from build123d import *

# Parameters (mm, degrees)
F1_DEPTH = 10
F2_SIZE  = 1
F3_R     = 1


with BuildPart() as f1:
    # F0 (on Top) → F1 (new body)
    with BuildSketch(Plane.XY):
        with BuildLine():
            Line((-2.507107, 0), (0, 0))
            Line((0, 0), (0, 1.35))
            ThreePointArc((0, 1.35), (-1.15, 2.5), (0, 3.65))
            Line((0, 3.65), (0, 8.907107))
            Line((0, 8.907107), (5.3, 8.907107))
            Line((5.3, 8.907107), (5.3, 3.607107))
            Line((5.3, 3.607107), (3.5, 3.607107))
            Line((3.5, 3.607107), (3.5, 1.607107))
            Line((3.5, 1.607107), (7.1, 1.607107))
            Line((7.1, 1.607107), (7.1, 10.707107))
            Line((7.1, 10.707107), (-1.8, 10.707107))
            Line((-1.8, 10.707107), (-1.8, 4.707107))
            Line((-1.8, 4.707107), (-2.507107, 4))
            Line((-2.507107, 4), (-2.507107, 0))
        make_face()
    extrude(amount=F1_DEPTH)

    # F2
    f2_edges = [f1.edges().sort_by_distance(p)[0] for p in [
        (-2.507107, 0, 5),
    ]]
    chamfer(f2_edges, length=F2_SIZE)

    # F3
    f3_edges = [f1.edges().sort_by_distance(p)[0] for p in [
        (7.1, 1.607107, 5),
        (7.1, 10.707107, 5),
        (-1.8, 10.707107, 5),
    ]]
    fillet(f3_edges, radius=F3_R)


solid = f1.part
Model file for the job. Use its own axes, mm. A direction names the side the tool comes from. Coordinates: 2 decimals unless noted, no trailing zeros. Order: outer loops, then holes, each group sorted by start corner. A loop starts at its lowest first (then second) coordinate and runs counter-clockwise, first axis right, second up. Notation, with made-up numbers: (8, 69.5) -> (26, 69.5) arc R20 cw to (26, 98.5) -> close; hole circle Ø11 at (-9, 65.25). An arc over 180 degrees is marked (long way). Return JSON: item names as keys, results as strings. Group by question number.
Item 1: Wall check: line 1 along Y through (x, z) = (4, 7.75); line 2 along Y through (x, z) = (1, 6.75); line 3 along X through (y, z) = (9.5, 1.5). Give the ranges that are in metal, low to high. Write a range as [from, to].
Item 2: Saw through at C-C on x = 5.5. Write the cut outline in (y, z).
Item 3: Flat gauge pins, fed straight in: P1, Ø1.5, axis at x = 3.5, z = 7.5, coming from the -Y side; P2, Ø1.6, axis at y = 7.5, z = 5, coming from the -X side; P3, Ø0.7, axis at y = 1, z = 2.5, coming from the +X side. Where does each tip first touch, or does it go through?
Item 4: Tool access for faces 1 (the flat face through (-1.8, 7, 5)), 2 (the flat face through (3.5, 3, 5)), 3 (the flat face through (-1, 0, 5)), 4 (the flat face through (0, 1, 5)), 5 (the flat face through (4, 3.607, 5)): list every direction of +Z, -Z, +X, -X, +Y, -Y with a clear straight run to the whole face (end or side of a thin tool).
Item 5: Saw through at A-A on x = 4.5. Write the cut outline in (y, z).
Item 6: Saw through at B-B on z = 8. Write the cut outline in (x, y), then the cut area to 4 significant figures.
Item 7: Pull direction Y, two halves, no side cores. Call faces 6 (the flat face through (3, 10.707, 5)), 7 (the flat face through (5.3, 6, 5)), 8 (the cylindrical face through (-1.15, 2.47, 4.93)), 9 (the flat face through (5, 1.607, 5)): pulls with the +Y half, pulls with the -Y half, needs draft (parallel to the pull), parting line crosses it, or undercut.
Item 8: Saw through at D-D on x = 3.25. Write the cut outline in (y, z).
Values found:
{
 "1": {"line 1": "y = [1.61, 3.61], [8.91, 10.71]", "line 2": "y = [8.91, 10.71]", "line 3": "x = [-1.8, 7.1]"},
 "2": {"outline": "(1.61, 0) -> (10.71, 0) -> (10.71, 10) -> (1.61, 10) -> close"},
 "3": {"P1": "stops at y = 1.61", "P2": "stops at x = -1.8", "P3": "stops at x = 0"},
 "4": {"face 1": "+Z, -Z, -X, +Y", "face 2": "+Z, -Z, -Y", "face 3": "+Z, -Z, +X, -X, -Y", "face 4": "+Z, -Z, +X, -Y", "face 5": "+Z, -Z"},
 "5": {"outline": "(1.61, 0) -> (3.61, 0) -> (3.61, 10) -> (1.61, 10) -> close; (8.91, 0) -> (10.71, 0) -> (10.71, 10) -> (8.91, 10) -> close"},
 "6": {"outline": "(-2.51, 1) -> (-1.51, 0) -> (0, 0) -> (0, 1.35) arc R1.15 cw to (0, 3.65) -> (0, 8.91) -> (5.3, 8.91) -> (5.3, 3.61) -> (3.5, 3.61) -> (3.5, 1.61) -> (6.1, 1.61) arc R1 ccw to (7.1, 2.61) -> (7.1, 9.71) arc R1 ccw to (6.1, 10.71) -> (-0.8, 10.71) arc R1 ccw to (-1.8, 9.71) -> (-1.8, 4.71) -> (-2.51, 4) -> close", "area": "48.65 mm2"},
 "7": {"face 6": "pulls with the +Y half", "face 7": "undercut", "face 8": "undercut", "face 9": "pulls with the -Y half"},
 "8": {"outline": "(8.91, 0) -> (10.71, 0) -> (10.71, 10) -> (8.91, 10) -> close"}
}
